from build123d import *

# Parameters (mm, degrees)
BOSS_EXTRUDE1_DEPTH = 5
SKETCH2_W           = 90
SKETCH2_H           = 2
CUT_EXTRUDE1_DEPTH  = 2


with BuildPart() as part:
    # Sketch1 → Boss-Extrude1 (new body)
    with BuildSketch(Plane(origin=(0, 0, 0), x_dir=(1, 0, 0), z_dir=(0, 1, 0))):
        Polygon((-27, 0), (0, 0), (0, 40), (-100, 40), (-100, 0), (-73, 0), (-73, 23), (-27, 23), align=None)
    extrude(amount=BOSS_EXTRUDE1_DEPTH)

    # Sketch2 → Cut-Extrude1 (cut)
    with BuildSketch(Plane(origin=(0, 5, 0), x_dir=(1, 0, 0), z_dir=(0, 1, 0))):
        Polygon((-100, 40), (-100, 0), (-95, 0), (-95, 38), (-95, 40), align=None)
        with Locations((-50, 39)):
            Rectangle(SKETCH2_W, SKETCH2_H)
        Polygon((-5, 40), (-5, 38), (-5, 0), (0, 0), (0, 40), align=None)
    extrude(amount=-CUT_EXTRUDE1_DEPTH, mode=Mode.SUBTRACT)


solid = part.part
Model file for the job. Use its own axes, mm. A direction names the side the tool comes from. Give positions to 0.01 mm unless a question says otherwise; leave off trailing zeros. Loops run counter-clockwise (first coordinate to the right, second up) from the corner with the lowest first, then second, coordinate; pieces in that order, holes last. Notation, with made-up numbers: (23, 72.25) -> (45, 72.25) arc R36 cw to (45, 111.25) -> close; hole circle Ø9 at (-33, -17). An arc over 180 degrees is marked (long way). Use a Markdown table: item, result. Add a question column.
(1) Slice it at D-D on z = -36.5. List the corners of the cut face in (x, y).
(2) Wall check: line 1 along X through (y, z) = (0.85, -5.5); line 2 along X through (y, z) = (3.3, -12); line 3 along Z through (x, y) = (-29.5, 3.75). Give the ranges that are in metal, low to high.
(3) Slice it at C-C on x = -53. List the corners of the cut face in (y, z).
(4) Slice it at B-B on y = 1.25. List the corners of the cut face in (x, z).
(5) Slice it at A-A on z = -12.5. List the corners of the cut face in (x, y).
(6) Drop flat-ended pins along their axis: pin 1 Ø0.6 at (y, z) = (4.5, -24.5) entering from -X; pin 2 Ø0.6 at (y, z) = (3.5, -10.5) entering from +X. Give the stop position or say it passes through.
(7) Mould opens along X. For faces 1 (the flat face through (-100, 1, -20)), 2 (the flat face through (-27, 2, -12)), 3 (the flat face through (-50.6, 5, -23.5)) say: +X half, -X half, draft (parallel to the pull), parting line (faces both ways), or undercut.
(8) Tool access for faces 4 (the flat face through (-51, 4, -38)), 5 (the flat face through (-5, 4, -19)), 6 (the flat face through (-95, 4, -19)), 7 (the flat face through (-73, 2, -11)), 8 (the flat face through (-49, 1, -40)): list every direction of +Z, -Z, +X, -X, +Y, -Y with a clear straight run to the whole face (end or side of a thin tool).
Filled sheet:
| question | item | result |
|---|---|---|
| 1 | outline | (-100, 0) -> (0, 0) -> (0, 3) -> (-5, 3) -> (-5, 5) -> (-95, 5) -> (-95, 3) -> (-100, 3) -> close |
| 2 | line 1 | -100 to -73, -27 to 0 |
| 2 | line 2 | -95 to -73, -27 to -5 |
| 2 | line 3 | -38 to -23 |
| 3 | outline | (0, -40) -> (3, -40) -> (3, -38) -> (5, -38) -> (5, -23) -> (0, -23) -> close |
| 4 | outline | (-100, -40) -> (0, -40) -> (0, 0) -> (-27, 0) -> (-27, -23) -> (-73, -23) -> (-73, 0) -> (-100, 0) -> close |
| 5 | outline | (-100, 0) -> (-73, 0) -> (-73, 5) -> (-95, 5) -> (-95, 3) -> (-100, 3) -> close; (-27, 0) -> (0, 0) -> (0, 3) -> (-5, 3) -> (-5, 5) -> (-27, 5) -> close |
| 6 | pin 1 | x = -95 |
| 6 | pin 2 | x = -5 |
| 7 | face 1 | -X half |
| 7 | face 2 | undercut |
| 7 | face 3 | draft |
| 8 | face 4 | -Z, +X, -X, +Y |
| 8 | face 5 | +Z, -Z, +X, +Y |
| 8 | face 6 | +Z, -Z, -X, +Y |
| 8 | face 7 | +Z, +Y, -Y |
| 8 | face 8 | -Z, +X, -X, +Y, -Y |
